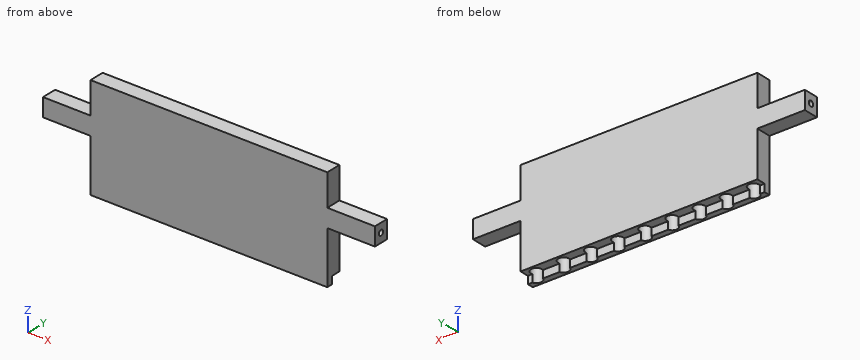
```python
from build123d import *

# Parameters (mm, degrees)
SKETCH_1_W          = 220
SKETCH_1_H          = 10
SKETCH_1_R          = 3.6
EXTRUDE_1_DEPTH     = 65
SKETCH_2_W          = 220
SKETCH_2_H          = 5
CUT_EXTRUDE_1_DEPTH = 6
SKETCH_3_W          = 31.511676707
SKETCH_3_H          = 35
SKETCH_3_H_2        = 18
SKETCH_3_W_2        = 31.571676707
CUT_EXTRUDE_2_DEPTH = 230.619250064
SKETCH_4_R          = 1.8
CUT_EXTRUDE_3_DEPTH = 10
CUT_EXTRUDE_START   = -10
SKETCH_5_R          = 1.8
CUT_EXTRUDE_4_DEPTH = 10
SKETCH_6_W          = 156.916646586
SKETCH_6_H          = 10
EXTRUDE_2_DEPTH     = 3


with BuildPart() as part:
    # Эскиз1 → Бобышка-Вытянуть1 (new body)
    with BuildSketch(Plane.XY):
        with Locations((110, 5)):
            Rectangle(SKETCH_1_W, SKETCH_1_H)
        with Locations((37.97, 5)):
            Circle(SKETCH_1_R, mode=Mode.SUBTRACT)
        with Locations((55.97, 5)):
            Circle(SKETCH_1_R, mode=Mode.SUBTRACT)
        with Locations((73.97, 5)):
            Circle(SKETCH_1_R, mode=Mode.SUBTRACT)
        with Locations((91.97, 5)):
            Circle(SKETCH_1_R, mode=Mode.SUBTRACT)
        with Locations((109.97, 5)):
            Circle(SKETCH_1_R, mode=Mode.SUBTRACT)
        with Locations((127.97, 5)):
            Circle(SKETCH_1_R, mode=Mode.SUBTRACT)
        with Locations((145.97, 5)):
            Circle(SKETCH_1_R, mode=Mode.SUBTRACT)
        with Locations((163.97, 5)):
            Circle(SKETCH_1_R, mode=Mode.SUBTRACT)
        with Locations((181.97, 5)):
            Circle(SKETCH_1_R, mode=Mode.SUBTRACT)
    extrude(amount=EXTRUDE_1_DEPTH)

    # Эскиз2 → Вырез-Вытянуть1 (cut)
    with BuildSketch(Plane(origin=(0, 10, 0), x_dir=(1, 0, 0), z_dir=(0, 1, 0))):
        with Locations((110, -2.5)):
            Rectangle(SKETCH_2_W, SKETCH_2_H)
    extrude(amount=-CUT_EXTRUDE_1_DEPTH, mode=Mode.SUBTRACT)

    # Эскиз3 → Вырез-Вытянуть2 (cut, through all)
    with BuildSketch(Plane(origin=(0, 10, 0), x_dir=(1, 0, 0), z_dir=(0, 1, 0))):
        with Locations((15.755838354, -17.5)):
            Rectangle(SKETCH_3_W, SKETCH_3_H)
        with Locations((15.755838354, -56)):
            Rectangle(SKETCH_3_W, SKETCH_3_H_2)
        with Locations((204.214161647, -17.5)):
            Rectangle(SKETCH_3_W_2, SKETCH_3_H)
        with Locations((204.214161647, -56)):
            Rectangle(SKETCH_3_W_2, SKETCH_3_H_2)
    extrude(amount=-CUT_EXTRUDE_2_DEPTH, mode=Mode.SUBTRACT)

    # Эскиз4 → Вырез-Вытянуть3 (cut)
    with BuildSketch(Plane.ZY):
        with Locations((41, 5)):
            Circle(SKETCH_4_R)
    extrude(amount=-CUT_EXTRUDE_3_DEPTH, mode=Mode.SUBTRACT)

    # Эскиз5 → Вырез-Вытянуть4 (cut)
    with BuildSketch(Plane(origin=(220, 0, 0), x_dir=(0, 0, -1), z_dir=(1, 0, 0)).offset(CUT_EXTRUDE_START)):
        with Locations(Location((-41, 5, 0), (0, 0, 180))):
            Circle(SKETCH_5_R)
    extrude(amount=CUT_EXTRUDE_4_DEPTH, mode=Mode.SUBTRACT)

    # Эскиз6 → Бобышка-Вытянуть2 (add)
    with BuildSketch(Plane.XY.offset(65)):
        with Locations((109.97, 5)):
            Rectangle(SKETCH_6_W, SKETCH_6_H)
    extrude(amount=EXTRUDE_2_DEPTH)


solid = part.part
```
Model file for the job. Use its own axes, mm. Coordinates: 2 decimals unless noted, no trailing zeros. Order: outer loops, then holes, each group sorted by start corner. A loop starts at its lowest first (then second) coordinate and runs counter-clockwise, first axis right, second up. Notation, with made-up numbers: (-28, 55) -> (31, 55) arc R13 ccw to (31, 60) -> close; hole circle Ø10 at (-19, 13.25). An arc over 180 degrees is marked (long way). Return JSON: item names as keys, results as strings.
Item 1: Slice it at B-B (x = 82). Write the cut outline in (y, z).
Model answer:
{"outline": "(0, 0) -> (4, 0) -> (4, 5) -> (10, 5) -> (10, 68) -> (0, 68) -> close"}
Item 2: Wall check: line 1 along Y through (x, z) = (145.97, 46); line 2 along Z through (x, y) = (217, 5); line 3 along Z through (x, y) = (170.5, 4.75). Give the ranges that are in metal, low to high. Write a range as from..to.
Model answer:
{"line 1": "y = 0..1.4, 8.6..10", "line 2": "z = 35..39.2, 42.8..47", "line 3": "z = 5..68"}
Item 3: Slice it at C-C (x = 16.5). Write the cut outline in (y, z).
Model answer:
{"outline": "(0, 35) -> (10, 35) -> (10, 47) -> (0, 47) -> close"}
Item 4: Pin check, flat tips, straight feed: P1, Ø3, axis at x = 203, y = 3.5, coming from the +Z side; P2, Ø6, axis at x = 93, y = 6, coming from the -Z side; P3, Ø1.5, axis at y = 4.5, z = 12.5, coming from the -X side. Stop position of each tip, or through.
Model answer:
{"P1": "stops at z = 47", "P2": "stops at z = 5", "P3": "stops at x = 31.51"}
Item 5: Slice it at A-A (z = 12.5). Count the separate pieces of the cut face and the enclosed holes in it, then the cut area to 3 significant figures.
Model answer:
{"separate pieces": "1", "enclosed holes": "9", "area": "1,200 mm²"}
